```python
from build123d import *

# Parameters (mm, degrees)
BOSS_EXTRUDE1_DEPTH                               = 6.35
CSK_FOR_6_FLAT_HEAD_MACHINE_SCREW_100_D           = 3.7973
CSK_FOR_6_FLAT_HEAD_MACHINE_SCREW_100_CSINK_D     = 7.0866
CSK_FOR_6_FLAT_HEAD_MACHINE_SCREW_100_CSINK_ANGLE = 100
CUT_EXTRUDE1_DEPTH                                = 85.302079601


with BuildPart() as part:
    # Sketch1 → Boss-Extrude1 (new body)
    with BuildSketch(Plane(origin=(0, 0, 0), x_dir=(0, 0, -1), z_dir=(1, 0, 0))):
        Polygon((76.2, 15.875), (41.275, 15.875), (41.275, 0), (76.2, 0), (76.2, 1.5875), (82.55, 1.5875), (82.55, 14.2875), (76.2, 14.2875), align=None)
        Polygon((41.275, 0), (41.275, 15.875), (6.35, 15.875), (6.35, 14.2875), (0, 14.2875), (0, 1.5875), (6.35, 1.5875), (6.35, 0), align=None)
    extrude(amount=BOSS_EXTRUDE1_DEPTH)

    # CSK for #6 Flat Head Machine Screw (100)1 (through all)
    with Locations(Plane.ZY):
        with Locations((-79.375, 7.9375), (-3.175, 7.9375)):
            CounterSinkHole(CSK_FOR_6_FLAT_HEAD_MACHINE_SCREW_100_D / 2, CSK_FOR_6_FLAT_HEAD_MACHINE_SCREW_100_CSINK_D / 2, counter_sink_angle=CSK_FOR_6_FLAT_HEAD_MACHINE_SCREW_100_CSINK_ANGLE)

    # Sketch4 → Cut-Extrude1 (cut, through all)
    with BuildSketch(Plane.ZY):
        Polygon((-49.83638683, 7.9375), (-73.025, 11.415791976), (-73.025, 4.459208024), align=None)
        Polygon((-18.08638683, 12.7), (-64.46361317, 12.7), (-41.275, 9.221708024), align=None)
        Polygon((-9.525, 11.415791976), (-32.71361317, 7.9375), (-9.525, 4.459208024), align=None)
        Polygon((-18.08638683, 3.175), (-41.275, 6.653291976), (-64.46361317, 3.175), align=None)
    extrude(amount=-CUT_EXTRUDE1_DEPTH, mode=Mode.SUBTRACT)


solid = part.part
```
Model file for the job. Use its own axes, mm. A direction names the side the tool comes from. Coordinates: 2 decimals unless noted, no trailing zeros. Order: outer loops, then holes, each group sorted by start corner. A loop starts at its lowest first (then second) coordinate and runs counter-clockwise, first axis right, second up. Notation, with made-up numbers: (45, 49) - (62, 49) arc R13 cw to (62, 73) - close; hole circle Ø11 at (25.5, 36). An arc over 180 degrees is marked (long way). Return JSON: item names as keys, results as strings. Group by question number.
1) Flat gauge pins, fed straight in: P1, Ø6, axis at y = 13, z = -17.5, coming from the -X side; P2, Ø3, axis at x = 2, z = -3, coming from the -Y side; P3, Ø0.8, axis at x = 3, y = 15.5, coming from the +Z side; P4, Ø4.5, axis at y = 7.94, z = -3.18, coming from the -X side. Where does each tip first touch, or does it go through?
2) Tool access for faces 1 (the flat face through (3, 8, -82.55)), 2 (the flat face through (3.131, 6.223, -21.282)), 3 (the flat face through (3, 14.288, -3)), 4 (the flat face through (3, 1.588, -79)): list every direction of +Z, -Z, +X, -X, +Y, -Y with a clear straight run to the whole face (end or side of a thin tool).
3) Saw through at B-B, the plane x = 2.75. Count the separate pieces of the cut face and the enclosed holes in it, plus the area to 3 significant figures.
4) Saw through at C-C, the plane z = -21. Write the cut outline in (x, y) (3 decimals), plus the area to 3 significant figures.
5) Saw through at A-A, the plane z = -38. Write the cut outline in (x, y) (3 decimals).
6) Probe line 1 (Y direction, x = 1.75, z = -47.5) (3 decimals); line 2 (Y direction, x = 2.5, z = -48) (3 decimals); line 3 (Y direction, x = 5.25, z = -56) (3 decimals). List the from-to ranges inside material, lowest first. Write a range as from..to.
7) Mould opens along Y. For faces 5 (the flat face through (3.131, 10.985, -53.032)), 6 (the flat face through (3, 1.588, -3)), 7 (the flat face through (3, 1, -76.2)) say: released by +Y, released by -Y, zero draft, split by the parting line, or undercut.
Values found:
{
 "1": {"P1": "stops at x = 0", "P2": "stops at y = 1.59", "P3": "stops at z = -6.35", "P4": "stops at x = 1.08"},
 "2": {"face 1": "-Z, +X, -X, +Y, -Y", "face 2": "+X, -X", "face 3": "+Z, +X, -X, +Y", "face 4": "-Z, +X, -X, -Y"},
 "3": {"separate pieces": "1", "enclosed holes": "6", "area": "925 mm²"},
 "4": {"outline": "(0, 0) - (6.35, 0) - (6.35, 3.175) - (0, 3.175) - close; (0, 3.612) - (6.35, 3.612) - (6.35, 6.18) - (0, 6.18) - close; (0, 9.695) - (6.35, 9.695) - (6.35, 12.263) - (0, 12.263) - close; (0, 12.7) - (6.35, 12.7) - (6.35, 15.875) - (0, 15.875) - close", "area": "72.9 mm²"},
 "5": {"outline": "(0, 0) - (6.35, 0) - (6.35, 3.175) - (0, 3.175) - close; (0, 6.162) - (6.35, 6.162) - (6.35, 9.713) - (0, 9.713) - close; (0, 12.7) - (6.35, 12.7) - (6.35, 15.875) - (0, 15.875) - close"},
 "6": {"line 1": "y = 0..3.175, 5.72..10.155, 12.7..15.875", "line 2": "y = 0..3.175, 5.645..10.23, 12.7..15.875", "line 3": "y = 0..3.175, 4.445..7.013, 8.862..11.43, 12.7..15.875"},
 "7": {"face 5": "undercut", "face 6": "released by -Y", "face 7": "zero draft"}
}
